Source: three-view drawing plus pictorial views. Frame: mm from the lowest corner of the part. Give positions to 0.01 mm unless a question says otherwise; leave off trailing zeros. Write each loop counter-clockwise with the first axis right and the second up, starting at its lowest first coordinate (ties: lowest second). Pieces come first, ordered by that corner, then holes.
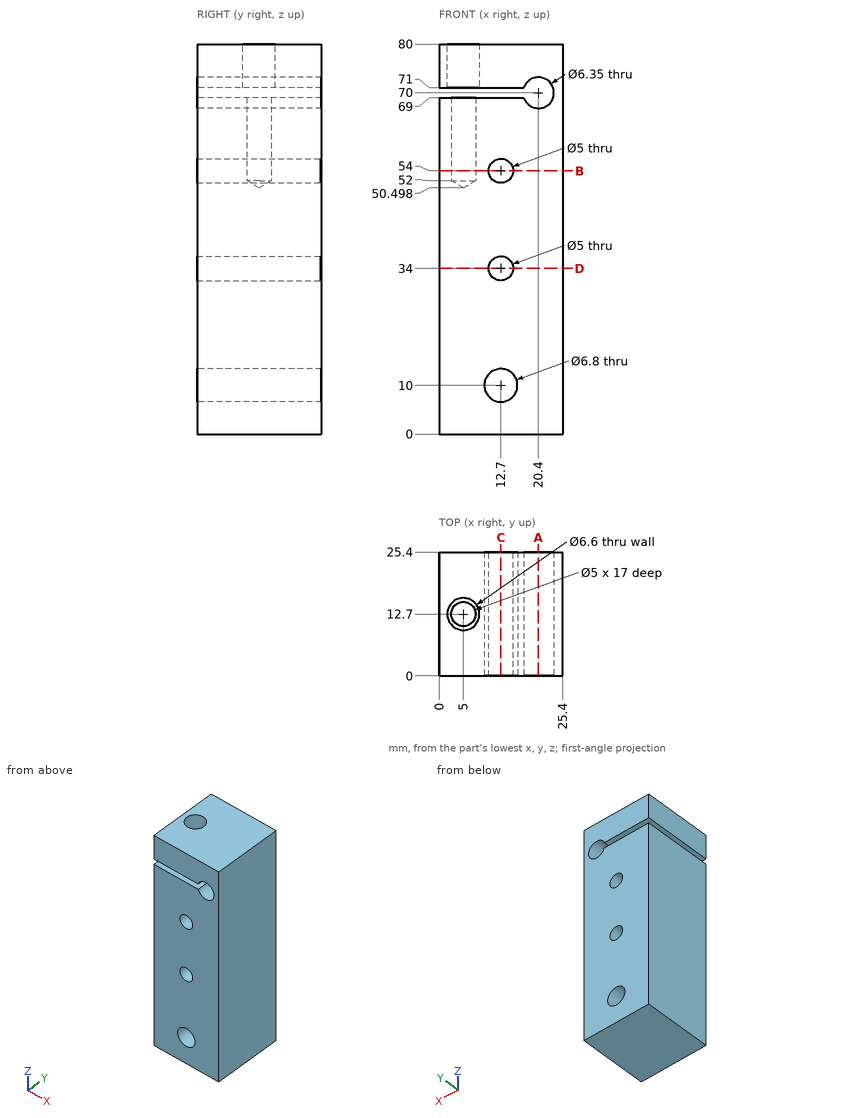
Q1. Section C-C on x = 12.7. Output: boundary loops of the cut face in (y, z), plus the area to 3 significant figures.
Filled sheet:
outline: (0, 0) - (25.4, 0) - (25.4, 6.6) - (0, 6.6) - close; (0, 13.4) - (25.4, 13.4) - (25.4, 31.5) - (0, 31.5) - close; (0, 36.5) - (25.4, 36.5) - (25.4, 51.5) - (0, 51.5) - close; (0, 56.5) - (25.4, 56.5) - (25.4, 69) - (0, 69) - close; (0, 71) - (25.4, 71) - (25.4, 80) - (0, 80) - close
area: 1,550 mm2
Q2. Ray query, line 1 along Z through (x, y) = (12.7, 9.5); line 2 along Y through (x, z) = (5, 74.75); line 3 along Y through (x, z) = (5, 58.25). Return the intervals inside material, ascending.
Filled sheet:
line 1: z = 0 to 6.6, 13.4 to 31.5, 36.5 to 51.5, 56.5 to 69, 71 to 80
line 2: y = 0 to 9.4, 16 to 25.4
line 3: y = 0 to 10.2, 15.2 to 25.4
Q3. Section D-D on z = 34. Output: boundary loops of the cut face in (x, y), plus the area to 3 significant figures.
Filled sheet:
outline: (0, 0) - (10.2, 0) - (10.2, 25.4) - (0, 25.4) - close; (15.2, 0) - (25.4, 0) - (25.4, 25.4) - (15.2, 25.4) - close
area: 518 mm2
Q4. Section A-A on x = 20.4. Output: boundary loops of the cut face in (y, z) (3 decimals), plus the area to 3 significant figures.
Filled sheet:
outline: (0, 0) - (25.4, 0) - (25.4, 66.825) - (0, 66.825) - close; (0, 73.175) - (25.4, 73.175) - (25.4, 80) - (0, 80) - close
area: 1,870 mm2
Q5. Pin query (flat end, axial travel): P1, Ø4, axis at x = 12.7, z = 10, coming from the -Y side; P2, Ø5, axis at x = 16, y = 21, coming from the -Z side. Return the tip coordinate at first contact, or that it passes through.
Filled sheet:
P1: passes through
P2: stops at z = 0
Q6. Section B-B on z = 54. Output: boundary loops of the cut face in (x, y).
Filled sheet:
outline: (0, 0) - (10.2, 0) - (10.2, 25.4) - (0, 25.4) - close; (15.2, 0) - (25.4, 0) - (25.4, 25.4) - (15.2, 25.4) - close; hole circle Ø5 at (5, 12.7)
